Build history of the part. All positions in model axes, mm. A direction names the side the tool comes from. Give positions to 0.01 mm unless a question says otherwise; leave off trailing zeros. Write each loop counter-clockwise with the first axis right and the second up, starting at its lowest first coordinate (ties: lowest second). Pieces come first, ordered by that corner, then holes.
Autodesk Inventor part; units mm, degrees
ref_plane "YZ Plane" through (0, 0, 0) normal (1, 0, 0) x (0, 1, 0)
ref_plane "XZ Plane" through (0, 0, 0) normal (0, 1, 0) x (-1, 0, 0)
ref_plane "XY Plane" through (0, 0, 0) normal (0, 0, 1) x (1, 0, 0)
sketch "Sketch1" plane through (0, 0, 0) normal (0, 0, 1) x (1, 0, 0)
  line L0 (-12.7, -25.4) -> (12.7, -25.4)
  line L1 (12.7, -25.4) -> (12.7, 25.4)
  line L2 (12.7, 25.4) -> (-12.7, 25.4)
  line L3 (-12.7, 25.4) -> (-12.7, -25.4)
  line L4 (-12.7, -25.4) -> (12.7, 25.4) construction
  line L5 (12.7, -25.4) -> (-12.7, 25.4) construction
  line L6 (-9.525, 22.225) -> (9.525, 22.225)
  line L7 (9.525, 22.225) -> (9.525, -22.225)
  line L8 (9.525, -22.225) -> (-9.525, -22.225)
  line L9 (-9.525, -22.225) -> (-9.525, 22.225)
  point P0 (0, 0)
  dimension "d0" = 25.4
  dimension "d1" = 50.8
  dimension "d2" = 3.175
extrude "Extrusion1" add sketch "Sketch1" along normal mid plane 914.4
sketch "Sketch2" plane through (-12.7, -25.4, 457.2) normal (0, -1, 0) x (1, 0, 0)
  line L0 (25.4, 0) -> (25.4, -914.4)
  line L1 (0, 0) -> (25.4, 0) construction
  line L2 (0, -914.4) -> (0, 0) construction
  line L3 (25.4, -914.4) -> (0, -914.4)
  line L4 (0, -914.4) -> (25.4, -889)
  point P0 (12.7, -457.2)
  dimension "d6" = 45
extrude "Extrusion2" cut sketch "Sketch2" against normal through all
sketch "Sketch4" plane through (-12.7, -25.4, 457.2) normal (0, -1, 0) x (1, 0, 0)
  line L0 (0, -914.4) -> (0, 0) construction
  point P0 (12.7, -457.2)
  point P1 (12.7, -889)
  point P2 (12.7, -876.3)
  point P3 (12.7, -863.6)
  point P4 (12.7, -850.9)
  point P5 (12.7, -838.2)
  dimension "d9" = 12.7
  dimension "d10" = 25.4
  dimension "d13" = 12.7
hole "Hole1" at (0, -25.4, -431.8) at (0, -25.4, -419.1) at (0, -25.4, -406.4) at (0, -25.4, -393.7) at (0, -25.4, -381) direction (0, 1, 0) diameter 5.1054 end through all
mirror "Mirror1" about plane through (0, 0, 0) normal (0, 0, 1) of "Hole1", "Extrusion2"
sketch "Sketch5" plane through (12.7, -25.4, -431.8) normal (1, 0, 0) x (0, 0, -1)
  line L0 (-431.8, 25.4) -> (-854.075, 25.4) construction
  dimension "d25" = 422.275
hole "Hole2" at (12.7, 0, 422.275) direction (-1, 0, 0) diameter 4.9784 end through all counterbore diameter 9.525 counterbore depth 12.7
sketch "Sketch6" plane through (-9.525, -22.225, -454.025) normal (1, 0, 0) x (0, 0, -1)
  circle A0 centre (-876.3, 22.225) radius 2.4892 construction
  line L0 (-876.3, 22.225) -> (-901.7, 22.225) construction
  line L1 (-901.7, 33.3375) -> (-901.7, 11.1125) construction
  point P0 (-454.025, 22.225)
  dimension "d33" = 25.4
  dimension "d34" = 22.225
hole "Hole3" at (-9.525, -11.1125, 447.675) at (-9.525, 11.1125, 447.675) direction (-1, 0, 0) diameter 4.9784 end through all
sketch "Sketch7" plane through (-12.7, -25.4, -457.2) normal (0, -1, 0) x (1, 0, 0)
  circle A0 centre (-4.7625, 885.825) radius 9.525
  line L0 (0, 0) -> (0, 914.4) construction
  point P0 (12.7, 457.2)
  dimension "d42" = 4.7625
  dimension "d43" = 28.575
  dimension "d44" = 19.05
extrude "Extrusion3" cut sketch "Sketch7" against normal blind 7.62
mirror "Mirror2" about plane through (0, 0, 0) normal (0, 1, 0) of "Extrusion3"
properties part number "TUBE,ELEVATOR,SIDE,STAGE1" material "Aluminum 6061 T6 0 Cold Formed"
(1) Drop flat-ended pins along their axis: pin 1 (6 mm diameter, centred on x = 0, z = -393.7, fed in from +Y); pin 2 (3.5 mm diameter, centred on x = -10.5, z = 430, fed in from +Y). Give the stop position or say it passes through.
(2) 3-axis set-ups, long thin cutter, end or side, ignore diameter. For faces 1 (the face through (10.4, 1.8, 434.1)), 2 (the face through (0, 22.225, -6)): which of +Z, -Z, +X, -X, +Y, -Y reach the whole face in a straight line?
(3) Probe line 1 (X direction, y = 22, z = 157.5) (3 decimals); line 2 (Y direction, x = 7, z = 258.5) (3 decimals); line 3 (X direction, y = 23.1, z = 393.7). List the from-to ranges inside material, lowest first.
(4) Saw through at A-A, the plane z = 285.5. List the corners of the cut face in (x, y) (3 decimals), plus the area to 3 significant figures.
(5) Mould opens along X. For faces 3 (the face through (12.7, 0, -6)), 4 (the face through (0, -25.4, -6)), 5 (the face through (0, -22.225, -6)) say: +X half, -X half, draft (parallel to the pull), parting line (faces both ways), or undercut.
Computed values:
1. pin 1: stops at y = 25.4
1. pin 2: stops at y = 17.78
2. face 1: +Z, +X, +Y, -Y
2. face 2: +Z, -Z
3. line 1: x = -12.7 to -9.525, 9.525 to 12.7
3. line 2: y = -25.4 to -22.225, 22.225 to 25.4
3. line 3: x = -12.7 to -2.55, 2.55 to 12.7
4. outline: (-12.7, -25.4) - (12.7, -25.4) - (12.7, 25.4) - (-12.7, 25.4) - close; hole (-9.525, -22.225) - (9.525, -22.225) - (9.525, 22.225) - (-9.525, 22.225) - close
4. area: 444 mm2
5. face 3: +X half
5. face 4: draft
5. face 5: undercut
